Build history of the part. All positions in model axes, mm. A direction names the side the tool comes from. Give positions to 0.01 mm unless a question says otherwise; leave off trailing zeros. Write each loop counter-clockwise with the first axis right and the second up, starting at its lowest first coordinate (ties: lowest second). Pieces come first, ordered by that corner, then holes.
from build123d import *

# Parameters (mm, degrees)
SKETCH1_R           = 8
SKETCH1_R_2         = 2.9
EXTRUDE1_DEPTH      = 10
EXTRUDE2_DEPTH      = 0.5
EXTRUDE2_DEPTH_BACK = 4
SKETCH4_W           = 5.227994408
SKETCH4_H           = 18.151774592
CUT_EXTRUDE1_DEPTH  = 104.897653244
FILLET4_R           = 14
SKETCH6_R           = 7.5
SKETCH6_R_2         = 2.726604726
EXTRUDE4_DEPTH      = 11
EXTRUDE6_DEPTH      = 3
EXTRUDE6_DEPTH_BACK = 13
SKETCH11_R          = 8.15177363
SKETCH11_R_2        = 4.885123956
EXTRUDE7_START      = 11
SKETCH8_R           = 7.5
SKETCH8_R_2         = 2.725
EXTRUDE7_DEPTH      = 11
FILLET19_R          = 3
FILLET23_R          = 5


with BuildPart() as part:
    # Sketch1 → Extrude1 (new body)
    with BuildSketch(Plane.XY):
        with Locations((12.741128877, -63.13435232)):
            Circle(SKETCH1_R)
        with Locations((12.741128877, -63.13435232)):
            Circle(SKETCH1_R_2, mode=Mode.SUBTRACT)
    extrude(amount=-EXTRUDE1_DEPTH)

    # Sketch2 → Extrude2 (add, two sides: drawn at the far end of the back side and taken through both)
    with BuildSketch(Plane(origin=(0, -71, 0), x_dir=(-1, 0, 0), z_dir=(0, 1, 0)).offset(-EXTRUDE2_DEPTH_BACK)):
        with BuildLine():
            Line((-12.741128877, 0), (12.908426363, 0))
            Line((12.908426363, 0), (12.908426363, -10))
            Line((12.908426363, -10), (-12.741128877, -10))
            Line((-12.741128877, -10), (-20.741128877, -10))
            Line((-20.741128877, -10), (-41.392249983, -30))
            Line((-41.392249983, -30), (-65.343112489, -30))
            Line((-65.343112489, -30), (-65.343112489, -19))
            Line((-65.343112489, -19), (-60.343112489, -19))
            ThreePointArc((-60.343112489, -19), (-45.681392415, -4.338279927), (-60.343112489, 10.323440147))
            Line((-60.343112489, 10.323440147), (-65.343112489, 10.323440147))
            Line((-65.343112489, 10.323440147), (-65.343112489, 21.323440147))
            Line((-65.343112489, 21.323440147), (-41.392249983, 21.323440147))
            Line((-41.392249983, 21.323440147), (-20.741128877, 0))
            Line((-20.741128877, 0), (-12.741128877, 0))
        make_face()
    extrude(amount=EXTRUDE2_DEPTH + EXTRUDE2_DEPTH_BACK)

    # Sketch4 → Cut-Extrude1 (cut, through all)
    with BuildSketch(Plane(origin=(0, 0, 0), x_dir=(0, 0, -1), z_dir=(1, 0, 0))):
        with Locations((4.605888128, -61.424112704)):
            Rectangle(SKETCH4_W, SKETCH4_H)
    extrude(amount=CUT_EXTRUDE1_DEPTH, mode=Mode.SUBTRACT)

    # Fillet4
    fillet4_edges = [part.edges().sort_by_distance(p)[0] for p in [
        (9.619072783, -70.5, -0.995945462),
        (15.863184971, -70.5, -8.609942666),
        (15.863184971, -70.5, -0.995945462),
        (9.619072783, -70.5, -8.609942666),
    ]]
    fillet(fillet4_edges, radius=FILLET4_R)

    # Sketch6 → Extrude4 (add)
    with BuildSketch(Plane.XY.offset(21.323440147)):
        with Locations((72.497656499, -72.75)):
            Circle(SKETCH6_R)
        with Locations((72.497656499, -72.75)):
            Circle(SKETCH6_R_2, mode=Mode.SUBTRACT)
    extrude(amount=-EXTRUDE4_DEPTH)

    # Sketch11 → Extrude6 (add, two sides: drawn at the far end of the back side and taken through both)
    with BuildSketch(Plane.XY.offset(-EXTRUDE6_DEPTH_BACK)):
        with Locations((-17.793550319, -71.960171152)):
            Circle(SKETCH11_R)
        with Locations((-17.793550319, -71.960171152)):
            Circle(SKETCH11_R_2, mode=Mode.SUBTRACT)
    extrude(amount=EXTRUDE6_DEPTH + EXTRUDE6_DEPTH_BACK)

    # Sketch8 → Extrude7 (add)
    with BuildSketch(Plane.XY.offset(-30).offset(EXTRUDE7_START)):
        with Locations((72.497656499, -72.75)):
            Circle(SKETCH8_R)
        with Locations((72.497656499, -72.75)):
            Circle(SKETCH8_R_2, mode=Mode.SUBTRACT)
    extrude(amount=-EXTRUDE7_DEPTH)

    # Fillet19
    fillet19_edges = [part.edges().sort_by_distance(p)[0] for p in [
        (65.343112489, -75, 15.823440147),
        (65.343112489, -75, -24.5),
        (65.343112489, -70.5, 15.823440147),
        (65.343112489, -70.5, -24.5),
    ]]
    fillet(fillet19_edges, radius=FILLET19_R)

    # Fillet23
    fillet23_edges = [part.edges().sort_by_distance(p)[0] for p in [
        (20.741128877, -68.378111591, -10),
        (20.741128877, -68.378111591, 0),
    ]]
    fillet(fillet23_edges, radius=FILLET23_R)


solid = part.part
(1) Probe line 1 (Z direction, x = 0, y = -68.75); line 2 (Z direction, x = 71.5, y = -76.5); line 3 (Y direction, x = 72.5, z = -27) (3 decimals). List the from-to ranges inside material, lowest first.
(2) Saw through at C-C, the plane z = 8. List the corners of the cut face in (x, y), plus the area to 3 significant figures.
(3) Saw through at B-B, the plane z = 17. List the corners of the cut face in (x, y).
(4) Saw through at D-D, the plane x = 38. List the corners of the cut face in (y, z).
(5) Saw through at A-A, the plane x = 12. List the corners of the cut face in (y, z), plus the area to 3 significant figures.
(6) 3-axis set-ups, long thin cutter, end or side, ignore diameter. For faces 1 (the face through (-12, -72, 3)), 2 (the face through (29.807, -72.152, 9.361)), 3 (the face through (12.4, -66.3, -1.992)), 4 (the face through (20.618, -68.197, -10.376)): which of +Z, -Z, +X, -X, +Y, -Y reach the whole face in a straight line?
(7) Drop flat-ended pins along their axis: pin 1 (5 mm diameter, centred on x = 37.5, y = -74, fed in from -Z); pin 2 (6.5 mm diameter, centred on x = 12.74, y = -63.13, fed in from -Z); pin 3 (7.5 mm diameter, centred on x = 12.74, y = -63.13, fed in from +Z). Give the stop position or say it passes through.
(8) Mould opens along X. For faces 5 (the face through (-0.062, -67.867, -8.59)), 6 (the face through (70, -74.3, 10.323)), 7 (the face through (12.883, -55.136, -8.729)) say: +X half, -X half, draft (parallel to the pull), parting line (faces both ways), or undercut.
Computed values:
1. line 1: z = -10 to -7.22, -1.99 to 0
1. line 2: z = -30 to -19, 10.32 to 21.32
1. line 3: y = -80.25 to -75.475, -70.025 to -65.25
2. outline: (28.49, -75) - (52.42, -75) - (52.42, -70.5) - (33.72, -70.5) arc R14 cw to (28.49, -69.49) - close
2. area: 109 mm2
3. outline: (37.21, -75) - (63.4, -75) arc R3 cw to (66, -76.5) arc R7.5 ccw (long way) to (66, -69) arc R3 cw to (63.4, -70.5) - (37.21, -70.5) - close; hole circle Ø5.45 at (72.5, -72.75)
4. outline: (-75, -26.71) - (-70.5, -26.71) - (-70.5, 17.82) - (-75, 17.82) - close
5. outline: (-75, -10) - (-65.94, -10) - (-65.94, -7.22) - (-70.5, -7.22) - (-70.5, -1.99) - (-65.94, -1.99) - (-65.94, 0) - (-75, 0) - close; (-60.33, -10) - (-55.17, -10) - (-55.17, -7.22) - (-60.33, -7.22) - close; (-60.33, -1.99) - (-55.17, -1.99) - (-55.17, 0) - (-60.33, 0) - close
5. area: 91.4 mm2
6. face 1: +Z, -X, +Y, -Y
6. face 2: +Z, +Y, -Y
6. face 3: +X, +Y
6. face 4: -Z, +Y, -Y
7. pin 1: stops at z = -28.65
7. pin 2: stops at z = -10
7. pin 3: stops at z = 0
8. face 5: undercut
8. face 6: draft
8. face 7: parting line
